Geometry: final body of the model. Coordinates: model frame, mm. A direction names the side the tool comes from. Give positions to 0.01 mm unless a question says otherwise; leave off trailing zeros. Write each loop counter-clockwise with the first axis right and the second up, starting at its lowest first coordinate (ties: lowest second). Pieces come first, ordered by that corner, then holes. Notation, with made-up numbers: M 23,38.25 L 37,38.25 A14 cw 37,53.25 Z; hole C -36,8 d5. An arc over 180 degrees is marked long. One line per question, with ' | ' between items.
from build123d import *

# Parameters (mm, degrees)
ESBO_O1_W                = 40
ESBO_O1_H                = 40
RESSALTO_EXTRUS_O1_DEPTH = 2
ESBO_O2_W                = 40
ESBO_O2_H                = 40
RESSALTO_EXTRUS_O2_DEPTH = 10
ESBO_O3_R                = 2.38
RESSALTO_EXTRUS_O3_DEPTH = 28.58


with BuildPart() as part:
    # Esboço1 → Ressalto-extrusão1 (new body)
    with BuildSketch(Plane(origin=(0, 0, 0), x_dir=(1, 0, 0), z_dir=(0, 1, 0))):
        with Locations((-15.012062533, -15.012062533)):
            Rectangle(ESBO_O1_W, ESBO_O1_H)
    extrude(amount=RESSALTO_EXTRUS_O1_DEPTH)

    # Esboço2 → Ressalto-extrusão2 (add)
    with BuildSketch(Plane.XZ):
        Polygon((-37.012062533, 37.012062533), (-37.012062533, 35.012062533), (-37.012062533, -6.987937467), (-35.012062533, -6.987937467), (6.987937467, -6.987937467), (6.987937467, -4.987937467), (6.987937467, 37.012062533), (4.987937467, 37.012062533), align=None)
        with Locations((-15.012062533, 15.012062533)):
            Rectangle(ESBO_O2_W, ESBO_O2_H, mode=Mode.SUBTRACT)
    extrude(amount=-RESSALTO_EXTRUS_O2_DEPTH)

    # Esboço3 → Ressalto-extrusão3 (add)
    with BuildSketch(Plane(origin=(0, 2, 0), x_dir=(1, 0, 0), z_dir=(0, 1, 0))):
        with Locations(Location((-15.012062533, -15.012062533, 0), (0, 0, 270))):
            Circle(ESBO_O3_R)
    extrude(amount=RESSALTO_EXTRUS_O3_DEPTH)


solid = part.part
(1) Cut plane D-D, the plane y = 23. Return loops of the section in (x, z).
Working result:
outline: C -15.01,15.01 d4.76
(2) First-contact query: P1, Ø2, axis at x = -5, z = 9.5, coming from the +Y side. Flat tip, straight axial feed; report the tip coordinate or a pass-through.
Working result:
P1: stops at y = 2
(3) Cut plane A-A, the plane y = 7.5. Return loops of the section in (x, z).
Working result:
outline: M -37.01,-6.99 L 6.99,-6.99 L 6.99,37.01 L -37.01,37.01 Z; C -15.01,15.01 d4.76; hole M -35.01,-4.99 L 4.99,-4.99 L 4.99,35.01 L -35.01,35.01 Z
(4) Set-up query: faces 1 (the face through (-16.46, 16.09, 13.123)), 2 (the face through (-37.012, 5, 15)). Return all of +Z, -Z, +X, -X, +Y, -Y with unobstructed straight access to the full face (end or side cutting, diameter ignored); none if empty.
Working result:
face 1: +Y | face 2: +Z, -Z, -X, +Y, -Y
(5) Material intervals for L1, parallel to Z at x = -5.5, y = 3; L2, parallel to X at y = 6.5, z = 30; L3, parallel to Y at x = -9, z = 11, sorted ascending. Write a range as [from, to].
Working result:
L1: z = [-6.99, -4.99], [35.01, 37.01] | L2: x = [-37.01, -35.01], [4.99, 6.99] | L3: y = [0, 2]
(6) Cut plane B-B, the plane z = 20.5. Return loops of the section in (x, y).
Working result:
outline: M -37.01,0 L 6.99,0 L 6.99,10 L 4.99,10 L 4.99,2 L -35.01,2 L -35.01,10 L -37.01,10 Z
(7) Cut plane C-C, the plane x = -28. Return loops of the section in (y, z), then the cut area to 3 significant figures.
Working result:
outline: M 0,-6.99 L 10,-6.99 L 10,-4.99 L 2,-4.99 L 2,35.01 L 10,35.01 L 10,37.01 L 0,37.01 Z | area: 120 mm^2
(8) Draft query along Z for faces 3 (the face through (-15, 5, 37.012)), 4 (the face through (4.988, 6, 15)), 5 (the face through (-15, 5, -6.988)), 6 (the face through (6.988, 5, 15)). Return one class per face: released by +Z, released by -Z, zero draft, split by the parting line, or undercut.
Working result:
face 3: released by +Z | face 4: undercut | face 5: released by -Z | face 6: zero draft
